Here's the drawing with two shaded views (mm, measured from the low corner). I have some questions. A direction names the side the tool comes from. Give positions to 0.01 mm unless a question says otherwise; leave off trailing zeros. Loops run counter-clockwise (first coordinate to the right, second up) from the corner with the lowest first, then second, coordinate; pieces in that order, holes last. Notation, with made-up numbers: (85.25, 66) - (109.25, 66) arc R21 cw to (109.25, 75) - close; hole circle Ø11 at (76.25, 20.5). An arc over 180 degrees is marked (long way). Use one line per item in the form item = value.
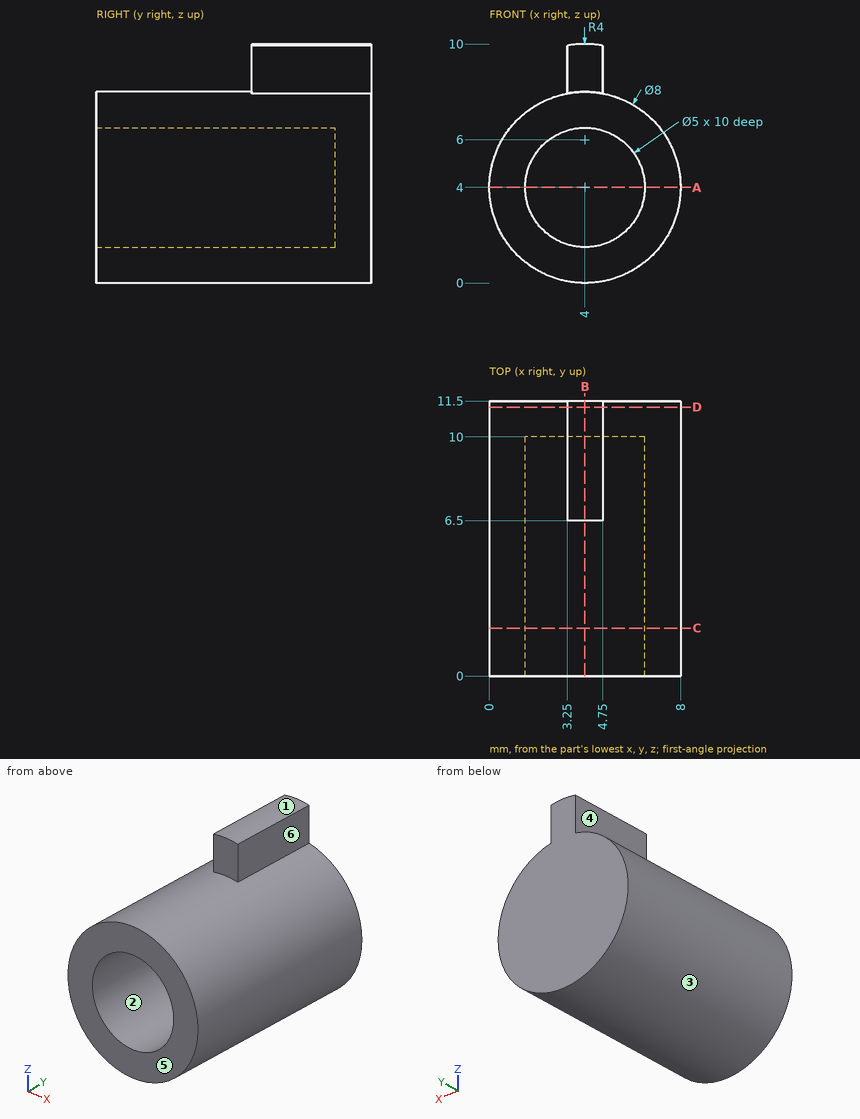
(1) If we section it at C-C (y = 2): List the corners of the cut face in (x, z) for me.
Geometry says:
outline = circle Ø8 at (4, 4); hole circle Ø5 at (4, 4)
(2) If we section it at B-B (x = 4): List the corners of the cut face in (y, z) for me, plus the area to 3 significant figures.
Geometry says:
outline = (0, 0) - (11.5, 0) - (11.5, 10) - (6.5, 10) - (6.5, 8) - (0, 8) - (0, 6.5) - (10, 6.5) - (10, 1.5) - (0, 1.5) - close
area = 52.0 mm²
(3) For P1, Ø1, axis at x = 1.5, y = 7, coming from the -Z side; P2, Ø4, axis at y = 4.5, z = 8.5, coming from the -X side; P3, Ø0.6, axis at y = 9.5, z = 9, coming from the +X side, each with a flat end and sliding along its axis, tell me the tip position at first contact or that it passes through.
Geometry says:
P1 = 0.54
P2 = 0.88
P3 = 4.75
(4) If we section it at A-A (z = 4): List the corners of the cut face in (x, y) for me.
Geometry says:
outline = (0, 0) - (1.5, 0) - (1.5, 10) - (6.5, 10) - (6.5, 0) - (8, 0) - (8, 11.5) - (0, 11.5) - close
(5) If we section it at D-D (y = 11.25): List the corners of the cut face in (x, z) for me, plus the area to 3 significant figures.
Geometry says:
outline = (3.25, 7.93) arc R4 ccw (long way) to (4.75, 7.93) - (4.75, 9.93) arc R4 ccw to (3.25, 9.93) - close
area = 53.3 mm²
(6) For the marked faces 5 and 6, which set-ups out of +Z, -Z, +X, -X, +Y, -Y let a thin tool reach every point of the face, with its end or its side?
Geometry says:
face_5 = +Z, -Z, +X, -X, -Y
face_6 = +Z, +X, +Y, -Y
(7) If I drill on probe 1 along Z at (x, y) = (4, 4); probe 2 along Z at (x, y) = (4, 8), over which ranges is the centre line in solid material (lowest first)?
Geometry says:
probe_1 = 0 to 1.5, 6.5 to 8
probe_2 = 0 to 1.5, 6.5 to 10
(8) Thinking about a two-plate mould opening in Z: for the marked faces 1, 2, 3 and 4, which applies, pulls with the +Z half, pulls with the -Z half, needs draft (parallel to the pull), parting line crosses it, or undercut?
Geometry says:
face_1 = pulls with the +Z half
face_2 = undercut
face_3 = parting line crosses it
face_4 = needs draft
